```python
from build123d import *

# Parameters (mm, degrees)
F0_W     = 127
F0_H     = 254
F0_R     = 3.175
F0_R_2   = 13.9954
F1_DEPTH = 6.35
F3_DEPTH = 63.5
F4_R     = 13.9954
F4_R_2   = 1.2446
F4_R_3   = 8.4963
F4_R_4   = 5.0038
F4_R_5   = 1.4986
F4_W     = 12.7
F4_H     = 50.8
F5_DEPTH = 12.7
F6_DEPTH = 2.0066
F7_DEPTH = 2.9972


with BuildPart() as f1:
    # F0 (on Front) → F1 (new body)
    with BuildSketch(Plane.XZ):
        Rectangle(F0_W, F0_H)
        with Locations((-38.1, -101.6)):
            Circle(F0_R, mode=Mode.SUBTRACT)
        with Locations((38.1, -101.6)):
            Circle(F0_R, mode=Mode.SUBTRACT)
        with Locations((-38.1, 101.6)):
            Circle(F0_R_2, mode=Mode.SUBTRACT)
        with Locations((38.1, 101.6)):
            Circle(F0_R, mode=Mode.SUBTRACT)
        with Locations((38.1, 101.6)):
            Circle(F0_R)
        with Locations((-38.1, -101.6)):
            Circle(F0_R)
    extrude(amount=F1_DEPTH)

    # F2 (on Right) → F3 (join, symmetric)
    with BuildSketch(Plane.YZ):
        with BuildLine():
            Line((44.638204, 82.55), (0, 82.55))
            Line((0, 82.55), (0, 76.2))
            Line((0, 76.2), (41.276354, 76.2))
            ThreePointArc((41.276354, 76.2), (43.553959, 75.237044), (44.45, 72.932292))
            Line((44.45, 72.932292), (41.660755, -22.550628))
            ThreePointArc((41.660755, -22.550628), (41.887722, -25.339829), (42.720032, -28.011611))
            Line((42.720032, -28.011611), (47.133445, -38.1))
            Line((47.133445, -38.1), (49.799549, -36.933647))
            Line((49.799549, -36.933647), (45.896387, -28.011611))
            ThreePointArc((45.896387, -28.011611), (45.064076, -25.339829), (44.837109, -22.550628))
            Line((44.837109, -22.550628), (47.81185, 79.282292))
            ThreePointArc((47.81185, 79.282292), (46.91581, 81.587044), (44.638204, 82.55))
        make_face()
    extrude(amount=F3_DEPTH, both=True)

    # F4 (on face) → F5 (join)
    with BuildSketch(Plane.XZ.offset(6.35)):
        with BuildLine():
            Line((-63.5, 57.605909), (-63.5, 73.201937))
            Line((-63.5, 73.201937), (-63.5, 127))
            Line((-63.5, 127), (5.894091, 127))
            ThreePointArc((5.894091, 127), (-74.021024, 137.521024), (-63.5, 57.605909))
        make_face()
        with BuildLine():
            Line((-63.5, 127), (-63.5, 73.201937))
            Line((-63.5, 73.201937), (-63.5, 57.605909))
            ThreePointArc((-63.5, 57.605909), (-12.7, 57.605909), (12.7, 101.6))
            ThreePointArc((12.7, 101.6), (10.969032, 114.748007), (5.894091, 127))
            Line((5.894091, 127), (-63.5, 127))
        make_face()
        with Locations((-38.1, 101.6)):
            Circle(F4_R, mode=Mode.SUBTRACT)
        with Locations((-38.1, 101.6)):
            Circle(F4_R)
        with Locations((-38.1, 90.6018)):
            Circle(F4_R_2, mode=Mode.SUBTRACT)
        with Locations((-49.0982, 101.6)):
            Circle(F4_R_2, mode=Mode.SUBTRACT)
        with Locations((-38.1, 101.6)):
            Circle(F4_R_3, mode=Mode.SUBTRACT)
        with Locations((-38.1, 112.5982)):
            Circle(F4_R_2, mode=Mode.SUBTRACT)
        with Locations((-27.1018, 101.6)):
            Circle(F4_R_2, mode=Mode.SUBTRACT)
        with Locations((-38.1, 101.6)):
            Circle(F4_R_3)
        with Locations((-38.1, 101.6)):
            Circle(F4_R_4, mode=Mode.SUBTRACT)
        with Locations((-38.1, 101.6)):
            Circle(F4_R_4)
        with Locations((-38.1, 101.6)):
            Circle(F4_R_5, mode=Mode.SUBTRACT)
        with Locations((3.175, -101.6)):
            Rectangle(F4_W, F4_H)
    extrude(amount=F5_DEPTH)

    # F4 (on face) → F6 (cut)
    with BuildSketch(Plane.XZ.offset(6.35)):
        with Locations((-38.1, 101.6)):
            Circle(F4_R_3)
        with Locations((-38.1, 101.6)):
            Circle(F4_R_4, mode=Mode.SUBTRACT)
        with Locations((-38.1, 101.6)):
            Circle(F4_R_4)
        with Locations((-38.1, 101.6)):
            Circle(F4_R_5, mode=Mode.SUBTRACT)
    extrude(amount=F6_DEPTH, mode=Mode.SUBTRACT)

    # F4 (on face) → F7 (cut)
    with BuildSketch(Plane.XZ.offset(6.35)):
        with Locations((-38.1, 101.6)):
            Circle(F4_R_4)
        with Locations((-38.1, 101.6)):
            Circle(F4_R_5, mode=Mode.SUBTRACT)
    extrude(amount=F7_DEPTH, mode=Mode.SUBTRACT)


solid = f1.part
```
Input: part model. Units: mm. Frame: model coordinates. A direction names the side the tool comes from. Give positions to 0.01 mm unless a question says otherwise; leave off trailing zeros. Order: outer loops, then holes, each group sorted by start corner. A loop starts at its lowest first (then second) coordinate and runs counter-clockwise, first axis right, second up. Notation, with made-up numbers: (6, -23) - (34, -23) arc R36 ccw to (34, 15) - close; hole circle Ø5 at (84.5, 72.5). An arc over 180 degrees is marked (long way). Use a Markdown table: item, result.
(1) Pin query (flat end, axial travel): pin 1 (7 mm diameter, centred on x = -15, y = -2, fed in from +Z); pin 2 (3 mm diameter, centred on x = -2.5, y = 25, fed in from +Z); pin 3 (3 mm diameter, centred on x = -38.1, z = 90.6, fed in from +Y); pin 4 (4 mm diameter, centred on x = 38.1, z = -101.6, fed in from +Y). Return the tip coordinate at first contact, or that it passes through.
Computed values:
| item | result |
|---|---|
| pin 1 | stops at z = 127 |
| pin 2 | stops at z = 82.55 |
| pin 3 | stops at y = -6.35 |
| pin 4 | passes through |
(2) Line query: line 1 (X direction, y = -8.65, z = 101.6); line 2 (Z direction, x = -38.1, y = -14.75); line 3 (Z direction, x = -38, y = -9). Output: solid intervals per line, ascending. Write a range as from..to.
Computed values:
| item | result |
|---|---|
| line 1 | x = -88.9..-50.34, -47.85..-43.1, -33.1..-28.35, -25.86..12.7 |
| line 2 | z = 50.8..89.36, 91.85..100.1, 103.1..111.35, 113.84..152.4 |
| line 3 | z = 50.8..89.36, 91.84..96.6, 106.6..111.36, 113.84..152.4 |
(3) Access query for faces 1 (the cylindrical face through (0.89, 45.07, -25.38)), 2 (the flat face through (-63.5, -1, -1)), 3 (the flat face through (-1, 0, 105)), 4 (the flat face through (-3.175, -13, -102)), 5 (the flat face through (1, 20, 76.2)). Directions: +Z, -Z, +X, -X, +Y, -Y. A direction counts if a zero-diameter tool reaches every point of the face in a straight line with its end or side. Return the directions, or none.
Computed values:
| item | result |
|---|---|
| face 1 | +X, -X, +Y |
| face 2 | +Z, -Z, -X, +Y |
| face 3 | +Z, +X, -X, +Y |
| face 4 | -Z, -X, -Y |
| face 5 | -Z, +X, -X |
(4) Section query B-B (z = -101.6). Output: boundary loops of the cut face in (x, y) (3 decimals).
Computed values:
| item | result |
|---|---|
| outline | (-63.5, -6.35) - (-3.175, -6.35) - (-3.175, -19.05) - (9.525, -19.05) - (9.525, -6.35) - (34.925, -6.35) - (34.925, 0) - (-63.5, 0) - close; (41.275, -6.35) - (63.5, -6.35) - (63.5, 0) - (41.275, 0) - close |
(5) Section query A-A (x = 38.1). Output: boundary loops of the cut face in (y, z) (3 decimals).
Computed values:
| item | result |
|---|---|
| outline | (-6.35, -127) - (0, -127) - (0, -104.775) - (-6.35, -104.775) - close; (-6.35, -98.425) - (0, -98.425) - (0, 76.2) - (41.276, 76.2) arc R3.175 cw to (44.45, 72.932) - (41.661, -22.551) arc R12.7 ccw to (42.72, -28.012) - (47.133, -38.1) - (49.8, -36.934) - (45.896, -28.012) arc R12.7 cw to (44.837, -22.551) - (47.812, 79.282) arc R3.175 ccw to (44.638, 82.55) - (0, 82.55) - (0, 127) - (-6.35, 127) - close |
(6) Draft query along Z for faces 6 (the flat face through (9.525, -13, -102)), 7 (the cylindrical face through (-33.327, -8.845, 103.103)), 8 (the flat face through (0.89, 44.9, -32.99)). Return one class per face: released by +Z, released by -Z, zero draft, split by the parting line, or undercut.
Computed values:
| item | result |
|---|---|
| face 6 | zero draft |
| face 7 | undercut |
| face 8 | released by -Z |
(7) Section query C-C (y = -3.5). Output: boundary loops of the cut face in (x, z) (3 decimals), then the cut area to 3 significant figures.
Computed values:
| item | result |
|---|---|
| outline | (-63.5, -127) - (63.5, -127) - (63.5, 127) - (-63.5, 127) - close; hole circle Ø27.991 at (-38.1, 101.6); hole circle Ø6.35 at (38.1, -101.6) |
| area | 31,600 mm2 |
(8) Section query D-D (y = 18). Output: boundary loops of the cut face in (x, z).
Computed values:
| item | result |
|---|---|
| outline | (-63.5, 76.2) - (63.5, 76.2) - (63.5, 82.55) - (-63.5, 82.55) - close |
